Input: part model. Units: mm. Frame: model coordinates. A direction names the side the tool comes from. Coordinates: 2 decimals unless noted, no trailing zeros. Write each loop counter-clockwise with the first axis right and the second up, starting at its lowest first coordinate (ties: lowest second). Pieces come first, ordered by that corner, then holes. Notation, with made-up numbers: (28.5, 59) - (64.5, 59) arc R21 cw to (64.5, 94) - close; hole circle Ø8 at (1, 31.5). An arc over 180 degrees is marked (long way). Put each result on its own line as item: value. Start each with the question number.
1. Pull-direction query (Y, two-part tool) for faces 1 (the flat face through (0.622, -136.667, -406.559)), 2 (the flat face through (-44.45, -167, -399)), 3 (the flat face through (0.622, -172.862, -395.968)), 4 (the cylindrical face through (38.19, -160.83, -394.84)); classes: released by +Y, released by -Y, zero draft, split by the parting line, or undercut.
2. Line query: line 1 (Y direction, x = -28.5, z = -279); line 2 (Y direction, x = -30.5, z = -408). Output: solid intervals per line, ascending.
3. Cut plane A-A, the plane x = -30. Return loops of the section in (y, z) (1 decimal).
4. Access query for faces 5 (the flat face through (31.75, -149, -399)), 6 (the flat face through (44.45, -167, -399)), 7 (the flat face through (-19.05, -152.8, -400.4)). Directions: +Z, -Z, +X, -X, +Y, -Y. A direction counts if a zero-diameter tool reaches every point of the face in a straight line with its end or side. Return the directions, or none.
5. Cut plane C-C, the plane z = -499.5. Return loops of the section in (x, y).
6. Pin query (flat end, axial travel): pin 1 (10 mm diameter, centred on x = 33, z = -660, fed in from +Y); pin 2 (12 mm diameter, centred on x = 28, z = -380, fed in from -Y); pin 3 (20.5 mm diameter, centred on y = -152.9, z = -395.19, fed in from -X); pin 4 (4 mm diameter, centred on x = -10, z = -235.5, fed in from +Y). Return the tip coordinate at first contact, or that it passes through.
7. Cut plane B-B, the plane y = -191. Return loops of the section in (x, z).
from build123d import *

# Parameters (mm, degrees)
F1_DEPTH       = 44.45
F1_DEPTH_BACK  = 44.45
F3_D           = 9.525
F3_DEPTH       = 31.75
F3_CBORE_D     = 15.875
F3_CBORE_DEPTH = 25.4
F5_D           = 9.525
F5_CBORE_D     = 15.875
F5_CBORE_DEPTH = 12.7


with BuildPart() as f1:
    # F0 (on Right) → F1 (new body, two sides)
    with BuildSketch(Plane.YZ) as f1_sk:
        Polygon((-4.600528, -23.008825), (-44.441384, -23.008825), (-304.928464, -779.518237), (-265.087608, -779.518237), align=None)
    extrude(amount=F1_DEPTH)
    extrude(f1_sk.sketch, amount=-F1_DEPTH_BACK)

    # F3
    with Locations(Plane(origin=(-44.45, 0, 0), x_dir=(0, -1, 0), z_dir=(-1, 0, 0))):
        with Locations((152.900278, -395.189479)):
            CounterBoreHole(F3_D / 2, F3_CBORE_D / 2, F3_CBORE_DEPTH, depth=F3_DEPTH)

    # F5 (through all)
    with Locations(Plane.YZ.offset(44.45)):
        with Locations((-152.900278, -395.189479)):
            CounterBoreHole(F5_D / 2, F5_CBORE_D / 2, F5_CBORE_DEPTH)


solid = f1.part
Report:
1. face 1: released by +Y
1. face 2: zero draft
1. face 3: released by -Y
1. face 4: undercut
2. line 1: y = -132.59 to -92.75
2. line 2: y = -177 to -137.16
3. outline: (-304.9, -779.5) - (-265.1, -779.5) - (-4.6, -23) - (-44.4, -23) - close; hole circle Ø15.9 at (-152.9, -395.2)
4. face 5: +X
4. face 6: +Z, -Z, +X, +Y, -Y
4. face 7: -X
5. outline: (-44.45, -208.51) - (44.45, -208.51) - (44.45, -168.67) - (-44.45, -168.67) - close
6. pin 1: stops at y = -222.21
6. pin 2: stops at y = -169.43
6. pin 3: stops at x = -44.45
6. pin 4: stops at y = -77.08
7. outline: (-44.45, -564.35) - (44.45, -564.35) - (44.45, -448.65) - (-44.45, -448.65) - close
